```python
from build123d import *

# Parameters (mm, degrees)
F0_W      = 25.4
F0_H      = 12.065
F0_W_2    = 15.24
F0_H_2    = 5.08
F1_DEPTH  = 101.6
F6_W      = 5.08
F6_H      = 10.16
F2_DEPTH  = 101.6
F3_W      = 6.985
F3_H      = 87.63
F7_DEPTH  = 25.4
F8_DEPTH  = 25.4
F9_R      = 2.54
F5_DEPTH  = 5.08
F11_DEPTH = 5.08


with BuildPart() as f1:
    # F0 (on Top) → F1 (new body)
    with BuildSketch(Plane.XY):
        with Locations((2.554662, -10.724223)):
            Rectangle(F0_W, F0_H)
        with Locations((2.554662, -9.136723)):
            Rectangle(F0_W_2, F0_H_2, mode=Mode.SUBTRACT)
    extrude(amount=F1_DEPTH)

    # F6 (on Top) → F2 (join, through all)
    with BuildSketch(Plane.XY):
        with Locations((-7.605338, -21.836723)):
            Rectangle(F6_W, F6_H)
        with Locations((12.714662, -21.836723)):
            Rectangle(F6_W, F6_H)
    extrude(amount=F2_DEPTH)

    # F3 (on face) → F7 (cut, through all)
    with BuildSketch(Plane.YZ.offset(15.254662)):
        with Locations((-8.184223, 57.785)):
            Rectangle(F3_W, F3_H)
    extrude(amount=-F7_DEPTH, mode=Mode.SUBTRACT)

    # F4 (on face) → F8 (cut, through all)
    with BuildSketch(Plane.YZ.offset(15.254662)):
        Polygon((-11.676723, 101.6), (-26.916723, 101.6), (-26.916723, 30.48), (-16.756723, 50.8), (-11.676723, 50.8), align=None)
    extrude(amount=-F8_DEPTH, mode=Mode.SUBTRACT)

    # F9 (on face) → F5 (cut, through all)
    with BuildSketch(Plane(origin=(0, -11.676723, 0), x_dir=(-1, 0, 0), z_dir=(0, 1, 0))):
        with Locations((-2.554662, 40.64)):
            Circle(F9_R)
        with Locations((-2.554662, 25.4)):
            Circle(F9_R)
    extrude(amount=-F5_DEPTH, mode=Mode.SUBTRACT)

    # F10 (on face) → F11 (cut, through all)
    with BuildSketch(Plane(origin=(0, -11.676723, 0), x_dir=(-1, 0, 0), z_dir=(0, 1, 0))):
        Polygon((-0.014662, 21.59), (-0.014662, 29.21), (-2.554662, 31.75), (-5.094662, 29.21), (-5.094662, 21.59), (-2.554662, 19.05), align=None)
        Polygon((-2.554662, 44.232102), (-4.350713, 42.436051), (-0.758611, 42.436051), align=None)
        Polygon((-0.758611, 38.843949), (-4.350713, 38.843949), (-2.554662, 37.047898), align=None)
    extrude(amount=-F11_DEPTH, mode=Mode.SUBTRACT)


solid = f1.part
```
Source: CAD feature listing. Evaluate the final solid. Frame: model axes, mm. A direction names the side the tool comes from. Round coordinates to 2 decimals unless told otherwise and drop trailing zeros. Loops run counter-clockwise (first coordinate to the right, second up) from the corner with the lowest first, then second, coordinate; pieces in that order, holes last.
(1) Section query C-C (z = 6). Output: boundary loops of the cut face in (x, y), and give its area (3 significant figures).
From the geometry:
outline: (-10.15, -26.92) - (-5.07, -26.92) - (-5.07, -16.76) - (10.17, -16.76) - (10.17, -26.92) - (15.25, -26.92) - (15.25, -4.69) - (-10.15, -4.69) - close; hole (-5.07, -11.68) - (10.17, -11.68) - (10.17, -6.6) - (-5.07, -6.6) - close
area: 332 mm2
(2) Section query B-B (x = -2). Output: boundary loops of the cut face in (y, z).
From the geometry:
outline: (-16.76, 0) - (-11.68, 0) - (-11.68, 50.8) - (-16.76, 50.8) - close; (-6.6, 0) - (-4.69, 0) - (-4.69, 13.97) - (-6.6, 13.97) - close
(3) Material intervals for probe 1 along Y at (x, z) = (2.25, 3); probe 2 along X at (y, z) = (-17.25, 18); probe 3 along Z at (x, y) = (4.75, -12), sorted ascending.
From the geometry:
probe 1: y = -16.76 to -11.68, -6.6 to -4.69
probe 2: x = -10.15 to -5.07, 10.17 to 15.25
probe 3: z = 0 to 21.25, 29.55 to 39.36, 41.92 to 50.8
(4) Section query A-A (z = 23). Output: boundary loops of the cut face in (x, y), and give its area (3 significant figures).
From the geometry:
outline: (-10.15, -26.92) - (-5.07, -26.92) - (-5.07, -16.76) - (0.01, -16.76) - (0.01, -11.68) - (-10.15, -11.68) - close; (5.09, -16.76) - (10.17, -16.76) - (10.17, -26.92) - (15.25, -26.92) - (15.25, -11.68) - (5.09, -11.68) - close
area: 206 mm2
(5) Access query for faces 5 (the flat face through (-5.065, -9, 7)), 6 (the flat face through (-5.065, -22, 19)), 7 (the flat face through (3.842, -14.181, 20.338)), 8 (the flat face through (3, -6, 13.97)). Directions: +Z, -Z, +X, -X, +Y, -Y. A direction counts if a zero-diameter tool reaches every point of the face in a straight line with its end or side. Return the directions, or none.
From the geometry:
face 5: +Z, -Z
face 6: +Z, -Z, -Y
face 7: +Y, -Y
face 8: +Z, +X, -X, +Y
(6) Contact query for flat-ended pins moving along their axis: pin 1 Ø4.5 at (x, z) = (4.5, 34.5) entering from -Y; pin 2 Ø12.5 at (x, z) = (3.5, 33) entering from +Y; pin 3 Ø2 at (x, y) = (3, -7) entering from +Z. Output: stop coordinate, or through.
From the geometry:
pin 1: stops at y = -16.76
pin 2: stops at y = -11.68
pin 3: stops at z = 13.97
(7) Pull-direction query (X, two-part tool) for faces 1 (the flat face through (-10.145, -18, 19)), 2 (the flat face through (15.255, -18, 19)), 3 (the flat face through (-8, -26.917, 15)), 4 (the cylindrical face through (0.015, -14.181, 40.612)); classes: +X half, -X half, draft (parallel to the pull), parting line (faces both ways), or undercut.
From the geometry:
face 1: -X half
face 2: +X half
face 3: draft
face 4: undercut
(8) Section query D-D (y = -8.25). Output: boundary loops of the cut face in (x, z).
From the geometry:
outline: (-10.15, 0) - (-5.07, 0) - (-5.07, 13.97) - (-10.15, 13.97) - close; (10.17, 0) - (15.25, 0) - (15.25, 13.97) - (10.17, 13.97) - close
